from build123d import *

# Parameters (mm, degrees)
SKETCH1_W           = 12.7
SKETCH1_H           = 139.7
BOSS_EXTRUDE1_DEPTH = 12.7
SKETCH2_W           = 63.5
SKETCH2_H           = 12.7
BOSS_EXTRUDE2_DEPTH = 12.7
SKETCH3_W           = 12.7
SKETCH3_H           = 88.9
BOSS_EXTRUDE3_DEPTH = 12.7
SKETCH6_R           = 1.778
CUT_EXTRUDE1_DEPTH  = 89.9
BOSS_EXTRUDE7_START = -19.05
BOSS_EXTRUDE7_DEPTH = 12.7
BOSS_EXTRUDE8_START = 44.45
BOSS_EXTRUDE8_DEPTH = 12.7


with BuildPart() as part:
    # Sketch1 → Boss-Extrude1 (new body)
    with BuildSketch(Plane.XY):
        with Locations((6.35, 69.85)):
            Rectangle(SKETCH1_W, SKETCH1_H)
    extrude(amount=BOSS_EXTRUDE1_DEPTH)

    # Sketch2 → Boss-Extrude2 (add)
    with BuildSketch(Plane.ZY):
        with Locations((-31.75, 6.35)):
            Rectangle(SKETCH2_W, SKETCH2_H)
    extrude(amount=-BOSS_EXTRUDE2_DEPTH)

    # Sketch3 → Boss-Extrude3 (add)
    with BuildSketch(Plane.ZY):
        with Locations((-69.85, 44.45)):
            Rectangle(SKETCH3_W, SKETCH3_H)
    extrude(amount=-BOSS_EXTRUDE3_DEPTH)

    # Sketch6 → Cut-Extrude1 (cut, through all)
    with BuildSketch(Plane.XY.offset(12.7)):
        with BuildLine():
            ThreePointArc((6.35, 131.572), (8.128, 133.35), (6.35, 135.128))
            Line((6.35, 135.128), (6.35, 131.572))
        make_face()
        with Locations((6.35, 112.7125)):
            Circle(SKETCH6_R)
        with Locations((6.35, 123.03125)):
            Circle(SKETCH6_R)
    extrude(amount=-CUT_EXTRUDE1_DEPTH, mode=Mode.SUBTRACT)

    # Sketch7 → Boss-Extrude7 (add)
    with BuildSketch(Plane.XY.offset(12.7).offset(BOSS_EXTRUDE7_START)):
        Polygon((0, 0), (-27.729644095, -26.128085241), (-15.029644095, -26.128085241), (12.7, 0), align=None)
    extrude(amount=-BOSS_EXTRUDE7_DEPTH)

    # Sketch10 → Boss-Extrude8 (add)
    with BuildSketch(Plane(origin=(0, 0, -19.05), x_dir=(-1, 0, 0), z_dir=(0, 0, -1)).offset(BOSS_EXTRUDE8_START)):
        Polygon((-12.7, 0), (15.029644095, -26.128085241), (27.729644095, -26.128085241), (0, 0), align=None)
    extrude(amount=BOSS_EXTRUDE8_DEPTH)


solid = part.part
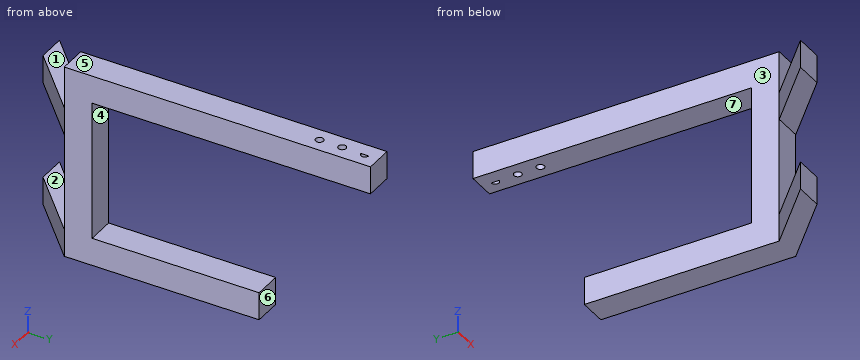
Could you check a few things on this model? Use its own coordinates, in mm. Face numbers are marked on the shaded views. A direction names the side the tool comes from. Give positions to 0.01 mm unless a question says otherwise; leave off trailing zeros. Order: outer loops, then holes, each group sorted by start corner. A loop starts at its lowest first (then second) coordinate and runs counter-clockwise, first axis right, second up. Notation, with made-up numbers: (17.25, 57) - (61.25, 57) arc R19 cw to (61.25, 93) - close; hole circle Ø1 at (76.5, -32.75). An arc over 180 degrees is marked (long way). Return JSON: item names as keys, results as strings. Group by question number.
Q1. Which directions (+Z, -Z, +X, -X, +Y, -Y) give clear straight access to the entire face, cutting with the end or side of a thin tool? Please do the marked faces 1, 2, 3 and 4.
Q2. Suppose I cut it at C-C, the plane z = -68. Please give me the cut outline in (x, y), and give its area (3 significant figures).
Q3. Please list where these lines run through material, in increasing order: line 1 along Y through (x, z) = (6, 6); line 2 along X through (y, z) = (84.5, -65.5); line 3 along X through (y, z) = (-11.5, -9.5). Write a range as [from, to].
Q4. Suppose I cut it at B-B, the plane x = -18.5. Please give me the cut outline in (y, z).
Q5. Suppose I cut it at A-A, the plane y = 133.35. Please give me the cut outline in (x, z), and give its area (3 significant figures).
Q6. Suppose I cut it at D-D, the plane y = 104. Please give me the cut outline in (x, z).
Q7. Will these pins go through, and if not, where does the flat tip stop? pin 1 Ø6.5 at (x, z) = (9, -36) entering from -Y; pin 2 Ø6.5 at (x, z) = (4, -41.5) entering from +Y; pin 3 Ø13 at (x, y) = (-6, -19) entering from +Z.
Q8. Thinking about a two-plate mould opening in Z: for the marked faces 5, 6 and 7, which applies, pulls with the +Z half, pulls with the -Z half, needs draft (parallel to the pull), parting line crosses it, or undercut?
Resolved:
{
 "1": {"face 1": "+Z, +X, -X, -Y", "face 2": "+X, -X, -Y", "face 3": "+Z, -Z, -X, +Y", "face 4": "+X, -X, +Y"},
 "2": {"outline": "(-27.73, -26.13) - (-15.03, -26.13) - (12.7, 0) - (12.7, 88.9) - (0, 88.9) - (0, 0) - close", "area": "1,460 mm2"},
 "3": {"line 1": "y = [0, 110.97], [114.46, 121.29], [124.77, 139.7]", "line 2": "x = [0, 12.7]", "line 3": "x = [-12.2, 0.5]"},
 "4": {"outline": "(-26.13, -76.2) - (-17.43, -76.2) - (-17.43, -63.5) - (-26.13, -63.5) - close; (-26.13, -19.05) - (-17.43, -19.05) - (-17.43, -6.35) - (-26.13, -6.35) - close"},
 "5": {"outline": "(0, 0) - (6.35, 0) - (6.35, 12.7) - (0, 12.7) - close; (8.13, 0) - (12.7, 0) - (12.7, 12.7) - (8.13, 12.7) - close", "area": "139 mm2"},
 "6": {"outline": "(0, 0) - (12.7, 0) - (12.7, 12.7) - (0, 12.7) - close"},
 "7": {"pin 1": "stops at y = 0", "pin 2": "stops at y = 12.7", "pin 3": "stops at z = -6.35"},
 "8": {"face 5": "pulls with the +Z half", "face 6": "needs draft", "face 7": "undercut"}
}
